Work out the finished part from the listing and answer in its coordinate system (mm). A direction names the side the tool comes from. Round coordinates to 2 decimals unless told otherwise and drop trailing zeros. Order: outer loops, then holes, each group sorted by start corner. A loop starts at its lowest first (then second) coordinate and runs counter-clockwise, first axis right, second up. Notation, with made-up numbers: (39.5, 66) - (76.5, 66) arc R27 cw to (76.5, 82) - close; hole circle Ø9 at (-21, 6.25). An arc over 180 degrees is marked (long way). Put each result on its own line as item: value.
```python
from build123d import *

# Parameters (mm, degrees)
F0_R     = 0.635
F1_DEPTH = 0.508
F2_DEPTH = 0.508
F3_R     = 0.762
F4_DEPTH = 25.4


with BuildPart() as f1:
    # F0 (on Front) → F1 (new body, symmetric)
    with BuildSketch(Plane.XZ):
        with BuildLine():
            Line((1.1718346045, 0.4895954042), (1.219972654, 0.352940113))
            ThreePointArc((1.219972654, 0.352940113), (1.1978539801, 0.4219547871), (1.1718346045, 0.4895954042))
        make_face()
        with BuildLine():
            ThreePointArc((0, 1.27), (0.7039580373, 1.0570445032), (1.1718346045, 0.4895954042))
            Line((1.1718346045, 0.4895954042), (0.59892699, 2.1159773936))
            ThreePointArc((0.59892699, 2.1159773936), (0.3669157635, 2.42326424), (0, 2.54))
            Line((0, 2.54), (0, 1.27))
        make_face()
        with BuildLine():
            ThreePointArc((0.762, -1.016), (1.1359225326, -0.5679612663), (1.27, 0))
            ThreePointArc((1.27, 0), (1.2574309664, 0.1782340166), (1.219972654, 0.352940113))
            Line((1.219972654, 0.352940113), (1.1718346045, 0.4895954042))
            ThreePointArc((1.1718346045, 0.4895954042), (0.7039580373, 1.0570445032), (0, 1.27))
            ThreePointArc((0, 1.27), (-1.2048277885, 0.4016092628), (-0.762, -1.016))
            ThreePointArc((-0.762, -1.016), (0, -1.27), (0.762, -1.016))
        make_face()
        Circle(F0_R, mode=Mode.SUBTRACT)
    extrude(amount=F1_DEPTH, both=True)

    # F0 (on Front) → F2 (join, symmetric)
    with BuildSketch(Plane.XZ):
        with BuildLine():
            Line((0.762, -2.159), (0.762, -1.016))
            ThreePointArc((0.762, -1.016), (0, -1.27), (-0.762, -1.016))
            Line((-0.762, -1.016), (-0.762, -2.159))
            Line((-0.762, -2.159), (0.762, -2.159))
        make_face()
    extrude(amount=F2_DEPTH, both=True)

    # F3 (on face) → F4 (join)
    with BuildSketch(Plane(origin=(0, 0, -2.159), x_dir=(1, 0, 0), z_dir=(0, 0, -1))):
        Circle(F3_R)
    extrude(amount=F4_DEPTH)


solid = f1.part
```
1) A cutting plane is placed at C-C on z = -22. Write down the section's boundary in (x, y), then the cut area to 3 significant figures.
Findings below:
outline: circle Ø1.52 at (0, 0)
area: 1.82 mm2
2) A cutting plane is placed at B-B on y = -0.25. Write down the section's boundary in (x, z) (3 decimals), then the cut area to 3 significant figures.
Findings below:
outline: (-0.762, -2.159) - (-0.72, -2.159) - (-0.72, -27.559) - (0.72, -27.559) - (0.72, -2.159) - (0.762, -2.159) - (0.762, -1.016) arc R1.27 ccw to (1.172, 0.49) - (0.599, 2.116) arc R0.635 ccw to (0, 2.54) - (0, 1.27) arc R1.27 ccw to (-0.762, -1.016) - close; hole circle Ø1.27 at (0, 0)
area: 42.8 mm2
3) For faces 1 (the cylindrical face through (-0.099, -0.756, -14.681)), 2 (the flat face through (0, 0, 2)), 3 (the flat face through (-1, 0.508, 0)), 4 (the flat face through (0.762, 0, -2)), determine the directions among +Z, -Z, +X, -X, +Y, -Y from which every point of the face is accessible in a straight line to the end or side of a thin tool.
Findings below:
face 1: -Z
face 2: +Z, -X, +Y, -Y
face 3: +Z, +X, -X, +Y
face 4: -Z, +X, +Y, -Y
4) A cutting plane is placed at A-A on z = 0. Write down the section's boundary in (x, y) (3 decimals), then the cut area to 3 significant figures.
Findings below:
outline: (-1.27, -0.508) - (-0.635, -0.508) - (-0.635, 0.508) - (-1.27, 0.508) - close; (0.635, -0.508) - (1.27, -0.508) - (1.27, 0.508) - (0.635, 0.508) - close
area: 1.29 mm2
5) Straight lines are drawn through the part: L1, parallel to X at y = 0.1, z = -17; L2, parallel to Y at x = -0.5, z = -18; L3, parallel to Z at x = 0.35, y = -0.2. For each, find the intervals that lie inside material, in ascending order. Write a range as from..to.
Findings below:
L1: x = -0.76..0.76
L2: y = -0.58..0.58
L3: z = -27.56..-0.53, 0.53..2.43
6) For a pull along X with two mould halves and no side action, classify faces 5 (the cylindrical face through (-0.08, 0.01, 0.63)), 6 (the flat face through (-0.762, 0, -2)), 7 (the flat face through (-1, -0.508, 0)), 8 (the flat face through (0.89, -0.01, 1.29)) as pulls with the +X half, pulls with the -X half, needs draft (parallel to the pull), parting line crosses it, or undercut.
Findings below:
face 5: undercut
face 6: pulls with the -X half
face 7: needs draft
face 8: pulls with the +X half
7) Given pin 1 Ø1.3 at (x, z) = (-0.5, -0.5) entering from +Y; pin 2 Ø1.3 at (x, z) = (0, -0.5) entering from -Y; pin 3 Ø0.8 at (y, z) = (0, -1.5) entering from +X, each flat-ended and moving along its own axis, determine where each tip first touches the part or whether it passes through.
Findings below:
pin 1: stops at y = 0.51
pin 2: stops at y = -0.51
pin 3: stops at x = 0.76
